```python
from build123d import *

# Parameters (mm, degrees)
EXTRUDE016_DEPTH = 60
BOX014_W         = 59
BOX014_H         = 60
BOX014_DEPTH     = 14.5


with BuildPart() as cpu_cooler_top:
    # Sketch001005021 (on Face4 of Box014) → Extrude016 (new body)
    with BuildSketch(Plane(origin=(44.5, -45.25, -18), x_dir=(-1, 0, 0), z_dir=(0, 1, 0))):
        Polygon((-45.25, 14.5), (-13.75, 14.5), (-16, 16.5), (-43, 16.5), align=None)
    extrude(amount=-EXTRUDE016_DEPTH)


with BuildPart() as cpu_cooler:
    # Box014 → Box014 (new body)
    with BuildSketch(Plane(origin=(44.5, -105.25, -18), x_dir=(1, 0, 0), z_dir=(0, 0, 1))):
        with Locations((29.5, 30)):
            Rectangle(BOX014_W, BOX014_H)
    extrude(amount=BOX014_DEPTH)

    # Fusion036: union CPU-Cooler-Top
    add(cpu_cooler_top.part)


solid = cpu_cooler.part
```
CAD build for the part. Positions are in the model's coordinates, mm. A direction names the side the tool comes from. Coordinates: 2 decimals unless noted, no trailing zeros. Write each loop counter-clockwise with the first axis right and the second up, starting at its lowest first coordinate (ties: lowest second). Pieces come first, ordered by that corner, then holes.
(1) Flat gauge pins, fed straight in: pin 1 (15 mm diameter, centred on x = 52, y = -89, fed in from +Z); pin 2 (4 mm diameter, centred on x = 97.5, y = -62, fed in from +Z). Where does each tip first touch, or does it go through?
(2) 3-axis set-ups, long thin cutter, end or side, ignore diameter. For faces 1 (the face through (51, -75, -3.5)), 2 (the face through (97, -75, -3.5)), 3 (the face through (44.5, -76, -11)): which of +Z, -Z, +X, -X, +Y, -Y reach the whole face in a straight line?
(3) Cut at B-B, the plane x = 52.5. List the corners of the cut face in (y, z), and give its area (3 significant figures).
(4) Cut at A-A, the plane y = -93. List the corners of the cut face in (x, z), and give its area (3 significant figures).
(5) Drill centre lines: probe 1 along Z at (x, y) = (97, -56); probe 2 along X at (y, z) = (-65.5, -3); probe 3 along X at (y, z) = (-67.5, -2.5) (3 decimals). Where is each one in solid material? Low to high.
Geometry says:
1. pin 1: stops at z = -2.39
1. pin 2: stops at z = -3.5
2. face 1: +Z, -X, +Y, -Y
2. face 2: +Z, +X, +Y, -Y
2. face 3: +Z, -Z, -X, +Y, -Y
3. outline: (-105.25, -18) - (-45.25, -18) - (-45.25, -3.5) - (-105.25, -3.5) - close
3. area: 870 mm2
4. outline: (44.5, -18) - (103.5, -18) - (103.5, -3.5) - (89.75, -3.5) - (87.5, -1.5) - (60.5, -1.5) - (58.25, -3.5) - (44.5, -3.5) - close
4. area: 914 mm2
5. probe 1: z = -18 to -3.5
5. probe 2: x = 58.81 to 89.19
5. probe 3: x = 59.375 to 88.625
